```python
from build123d import *

# Parameters (mm, degrees)
F0_R            = 22.5
F0_R_2          = 10
F1_DEPTH        = 20
F2_SIZE         = 1
F10_D           = 6.8
F10_DEPTH       = 15
F10_TIP         = 2.0429261047
F10_ON_F7_D     = 6.8
F10_ON_F7_DEPTH = 15
F10_ON_F7_TIP   = 2.0429261047
F10_ON_F9_D     = 6.8
F10_ON_F9_DEPTH = 15
F10_ON_F9_TIP   = 2.0429261047


with BuildPart() as f1:
    # F0 (on Top) → F1 (new body, symmetric)
    with BuildSketch(Plane.XY):
        Circle(F0_R)
        Circle(F0_R_2, mode=Mode.SUBTRACT)
    extrude(amount=F1_DEPTH, both=True)

    # F2
    f2_edges = [f1.edges().sort_by_distance(p)[0] for p in [
        (-22.5, 0, 20),
        (-22.5, 0, -20),
        (-10, 0, 20),
        (-10, 0, -20),
    ]]
    chamfer(f2_edges, length=F2_SIZE)

    # F10
    with Locations(Plane(origin=(11.25, -19.4855715851, 0), x_dir=(0.8660254038, 0.5, 0), z_dir=(0.5, -0.8660254038, 0))):
        with Locations((0, 0)):
            Hole(F10_D / 2, depth=F10_DEPTH)
            with Locations((0, 0, -(F10_DEPTH + F10_TIP / 2))):  # 118° drill point
                Cone(0, F10_D / 2, F10_TIP, mode=Mode.SUBTRACT)

    # F10 on F7
    with Locations(Plane(origin=(11.3809796361, 19.7124349697, 0), x_dir=(-0.8660254038, 0.5, 0), z_dir=(0.5, 0.8660254038, 0))):
        with Locations((0, 0)):
            Hole(F10_ON_F7_D / 2, depth=F10_ON_F7_DEPTH)
            with Locations((0, 0, -(F10_ON_F7_DEPTH + F10_ON_F7_TIP / 2))):  # 118° drill point
                Cone(0, F10_ON_F7_D / 2, F10_ON_F7_TIP, mode=Mode.SUBTRACT)

    # F10 on F9
    with Locations(Plane(origin=(-22.5, 0, 0), x_dir=(0, -1, 0), z_dir=(-1, 0, 0))):
        with Locations((0, 0)):
            Hole(F10_ON_F9_D / 2, depth=F10_ON_F9_DEPTH)
            with Locations((0, 0, -(F10_ON_F9_DEPTH + F10_ON_F9_TIP / 2))):  # 118° drill point
                Cone(0, F10_ON_F9_D / 2, F10_ON_F9_TIP, mode=Mode.SUBTRACT)


solid = f1.part
```
Model file for the job. Use its own axes, mm. A direction names the side the tool comes from. Give positions to 0.01 mm unless a question says otherwise; leave off trailing zeros. Order: outer loops, then holes, each group sorted by start corner. A loop starts at its lowest first (then second) coordinate and runs counter-clockwise, first axis right, second up.
1) Mould opens along Y. For faces 3 (the cylindrical face through (-4.878, -21.965, 0.266)), 4 (the cylindrical face through (10.27, -12.39, -2.07)), 5 (the flat face through (-5, 10, 20)) say: +Y half, -Y half, draft (parallel to the pull), parting line (faces both ways), or undercut.
2) Saw through at C-C, the plane z = 0. Write the cut outline in (x, y).
3) 3-axis set-ups, long thin cutter, end or side, ignore diameter. For faces 1 (the flat face through (-5, 10, -20)), 2 (the cylindrical face through (-15.86, -0.74, -3.32)): which of +Z, -Z, +X, -X, +Y, -Y reach the whole face in a straight line?
4) Pin check, flat tips, straight feed: pin 1 (5 mm diameter, centred on x = -11, z = 9, fed in from -Y); pin 2 (1 mm diameter, centred on y = 6, z = 2, fed in from -X); pin 3 (6 mm diameter, centred on x = 8.5, z = 7, fed in from -Y). Stop position of each tip, or through.
5) Wall check: probe 1 along Y at (x, z) = (0, 3.5); probe 2 along X at (y, z) = (0, -2). Give the ranges that are in metal, low to high.
6) Saw through at D-D, the plane z = -14.5. Write the cut outline in (x, y), then the cut area to 3 significant figures.
7) Saw through at A-A, the plane x = 0. Write the cut outline in (y, z), then the cut area to 3 significant figures.
8) Saw through at B-B, the plane y = 0. Write the cut outline in (x, z).
Computed:
1. face 3: parting line
1. face 4: undercut
1. face 5: draft
2. outline: (-22.24, -3.4) arc R22.5 ccw to (8.18, -20.96) - (1.76, -9.84) arc R10 cw to (-9.4, -3.4) - close; (-22.24, 3.4) - (-9.4, 3.4) arc R10 cw to (1.76, 9.84) - (8.18, 20.96) arc R22.5 ccw to start; (7.65, -6.44) - (14.07, -17.56) arc R22.5 ccw to (14.07, 17.56) - (7.65, 6.44) arc R10 cw to start
3. face 1: -Z, +X, -X, +Y, -Y
3. face 2: -X
4. pin 1: stops at y = -20.83
4. pin 2: stops at x = -21.82
4. pin 3: stops at y = -21.82
5. probe 1: y = -22.5 to -10, 10 to 22.5
5. probe 2: x = 10 to 22.5
6. outline: circle Ø45 at (0, 0); hole circle Ø20 at (0, 0)
6. area: 1,280 mm2
7. outline: (-22.5, -19) - (-21.5, -20) - (-11, -20) - (-10, -19) - (-10, 19) - (-11, 20) - (-21.5, 20) - (-22.5, 19) - close; (10, -19) - (11, -20) - (21.5, -20) - (22.5, -19) - (22.5, 19) - (21.5, 20) - (11, 20) - (10, 19) - close
7. area: 996 mm2
8. outline: (-22.5, -19) - (-21.5, -20) - (-11, -20) - (-10, -19) - (-10, -3.4) - (-22.5, -3.4) - close; (-22.5, 3.4) - (-10, 3.4) - (-10, 19) - (-11, 20) - (-21.5, 20) - (-22.5, 19) - close; (10, -19) - (11, -20) - (21.5, -20) - (22.5, -19) - (22.5, 19) - (21.5, 20) - (11, 20) - (10, 19) - close
